Geometry: see drawing. Coordinates: mm, zero at the bounding-box minimum. Round coordinates to 2 decimals unless told otherwise and drop trailing zeros. Order: outer loops, then holes, each group sorted by start corner. A loop starts at its lowest first (then second) coordinate and runs counter-clockwise, first axis right, second up. Notation, with made-up numbers: (15.5, 1.25) -> (62.5, 1.25) arc R17 ccw to (62.5, 24.25) -> close; hole circle Ø6 at (70.5, -12.75). An arc over 180 degrees is marked (long way). Use a Markdown table: item, result.
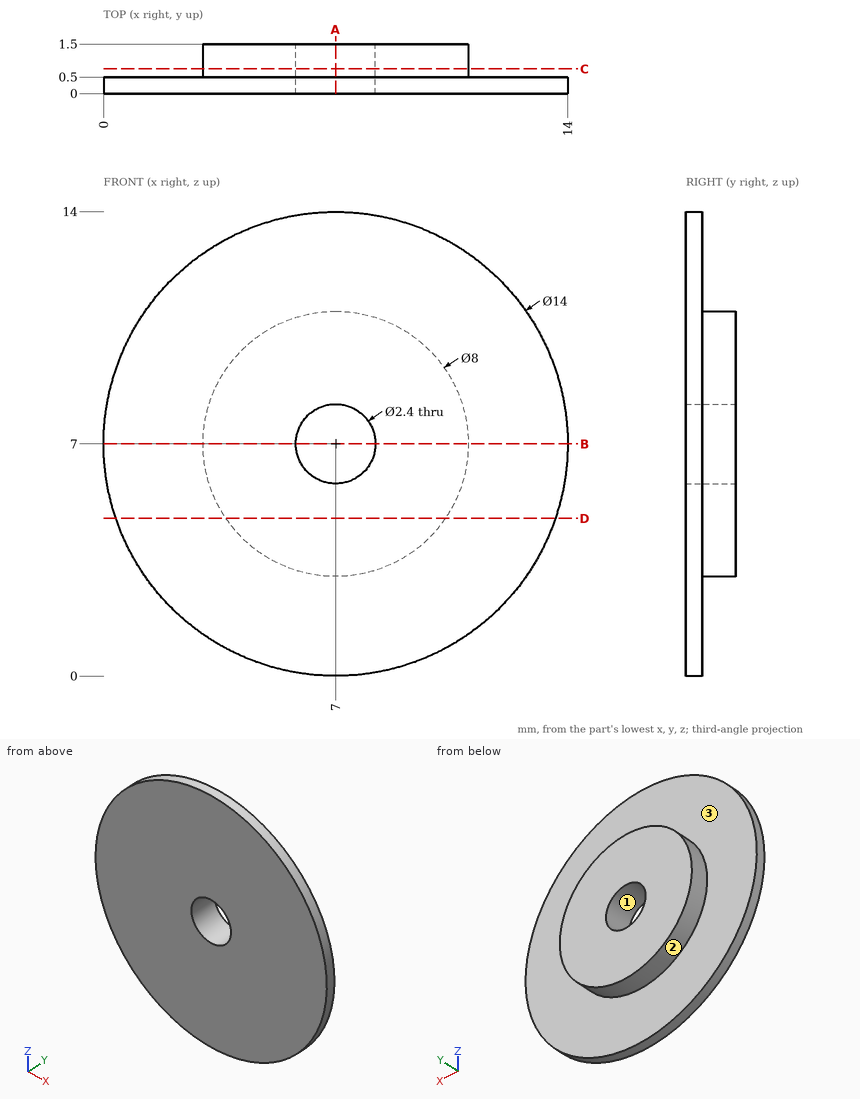
1) Cut plane D-D on z = 4.75. Return loops of the section in (x, y).
Answer key:
| item | result |
|---|---|
| outline | (0.37, 0) -> (13.63, 0) -> (13.63, 0.5) -> (10.31, 0.5) -> (10.31, 1.5) -> (3.69, 1.5) -> (3.69, 0.5) -> (0.37, 0.5) -> close |
2) Ray query, probe 1 along X at (y, z) = (0.75, 7); probe 2 along Y at (x, z) = (8.75, 12.75); probe 3 along X at (y, z) = (0.4, 7.75). Return the intervals inside material, ascending.
Answer key:
| item | result |
|---|---|
| probe 1 | x = 3 to 5.8, 8.2 to 11 |
| probe 2 | y = 0 to 0.5 |
| probe 3 | x = 0.04 to 6.06, 7.94 to 13.96 |
3) Cut plane C-C on y = 0.75. Return loops of the section in (x, z), and give its area (3 significant figures).
Answer key:
| item | result |
|---|---|
| outline | circle Ø8 at (7, 7); hole circle Ø2.4 at (7, 7) |
| area | 45.7 mm^2 |
4) Draft query along Z for the marked faces 1, 2 and 3. Return one class per face: released by +Z, released by -Z, zero draft, split by the parting line, or undercut.
Answer key:
| item | result |
|---|---|
| face 1 | undercut |
| face 2 | split by the parting line |
| face 3 | zero draft |
5) Contact query for a flat-ended pin moving along its axis: P1, Ø2, axis at x = 7, z = 7, coming from the -Y side. Output: stop coordinate, or through.
Answer key:
| item | result |
|---|---|
| P1 | passes through |
6) Cut plane A-A on x = 7. Return loops of the section in (y, z).
Answer key:
| item | result |
|---|---|
| outline | (0, 0) -> (0.5, 0) -> (0.5, 3) -> (1.5, 3) -> (1.5, 5.8) -> (0, 5.8) -> close; (0, 8.2) -> (1.5, 8.2) -> (1.5, 11) -> (0.5, 11) -> (0.5, 14) -> (0, 14) -> close |
7) Cut plane B-B on z = 7. Return loops of the section in (x, y).
Answer key:
| item | result |
|---|---|
| outline | (0, 0) -> (5.8, 0) -> (5.8, 1.5) -> (3, 1.5) -> (3, 0.5) -> (0, 0.5) -> close; (8.2, 0) -> (14, 0) -> (14, 0.5) -> (11, 0.5) -> (11, 1.5) -> (8.2, 1.5) -> close |
